from build123d import *

# Parameters (mm, degrees)
F1_R     = 2.5
F2_DEPTH = 7
F3_DEPTH = 2


with BuildPart() as f2:
    # F1 (on offset) → F2 (new body)
    with BuildSketch(Plane.XY):
        with Locations((-11.065031, 13.209959)):
            Circle(F1_R)
    extrude(amount=F2_DEPTH)

    # F1 (on offset) → F3 (join)
    with BuildSketch(Plane.XY):
        with BuildLine():
            ThreePointArc((-11.065031, 17.209959), (-13.893458, 16.038386), (-15.065031, 13.209959))
            Line((-15.065031, 13.209959), (-15.065031, -43.790041))
            ThreePointArc((-15.065031, -43.790041), (-13.893458, -46.618468), (-11.065031, -47.790041))
            ThreePointArc((-11.065031, -47.790041), (-8.236604, -46.618468), (-7.065031, -43.790041))
            Line((-7.065031, -43.790041), (-7.065031, 13.209959))
            ThreePointArc((-7.065031, 13.209959), (-8.236604, 16.038386), (-11.065031, 17.209959))
        make_face()
        with Locations((-11.065031, 13.209959)):
            Circle(F1_R, mode=Mode.SUBTRACT)
    extrude(amount=F3_DEPTH)


solid = f2.part
Source: CAD feature listing. Evaluate the final solid. Frame: model axes, mm. A direction names the side the tool comes from. Give positions to 0.01 mm unless a question says otherwise; leave off trailing zeros. Loops run counter-clockwise (first coordinate to the right, second up) from the corner with the lowest first, then second, coordinate; pieces in that order, holes last. Notation, with made-up numbers: (82.25, 29) -> (129.25, 29) arc R20 cw to (129.25, 40) -> close; hole circle Ø10 at (40.25, 17.25). An arc over 180 degrees is marked (long way). Use a Markdown table: item, result. Add a question column.
1) Section query D-D, the plane x = -8. Return the cut outline in (y, z).
2) Section query B-B, the plane x = -12.5. Return the cut outline in (y, z).
3) Reachability of faces 1 (the face through (-12.908, 14.9, 4.465)), 2 (the face through (-15.065, -15, 1)) from +Z, -Z, +X, -X, +Y, -Y: full face, straight path, thin tool, end or side. Return the list, or none.
4) Section query A-A, the plane z = 1. Return the cut outline in (x, y).
5) Section query C-C, the plane y = -33. Return the cut outline in (x, z), then the cut area to 3 significant figures.
6) First-contact query: pin 1 (4 mm diameter, centred on x = -14, y = -17.5, fed in from +Z); pin 2 (1.5 mm diameter, centred on x = -12.5, z = 3.5, fed in from -Y). Flat tips, straight axial feed; report the tip coordinate or a pass-through.
7) Line query: line 1 along Z through (x, y) = (-13.75, -9); line 2 along Y through (x, z) = (-12, 3); line 3 along Y through (x, z) = (-12.25, 4.25). Output: solid intervals per line, ascending. Write a range as [from, to].
Numbers:
| question | item | result |
|---|---|---|
| 1 | outline | (-46.36, 0) -> (15.78, 0) -> (15.78, 2) -> (-46.36, 2) -> close |
| 2 | outline | (-47.52, 0) -> (16.94, 0) -> (16.94, 2) -> (15.26, 2) -> (15.26, 7) -> (11.16, 7) -> (11.16, 2) -> (-47.52, 2) -> close |
| 3 | face 1 | +Z |
| 3 | face 2 | +Z, -Z, -X, +Y, -Y |
| 4 | outline | (-15.07, -43.79) arc R4 ccw to (-7.07, -43.79) -> (-7.07, 13.21) arc R4 ccw to (-15.07, 13.21) -> close |
| 5 | outline | (-15.07, 0) -> (-7.07, 0) -> (-7.07, 2) -> (-15.07, 2) -> close |
| 5 | area | 16.0 mm2 |
| 6 | pin 1 | stops at z = 2 |
| 6 | pin 2 | stops at y = 10.81 |
| 7 | line 1 | z = [0, 2] |
| 7 | line 2 | y = [10.89, 15.53] |
| 7 | line 3 | y = [11.01, 15.41] |
